from build123d import *

# Parameters (mm, degrees)
SKETCH2_W          = 40.136410409
SKETCH2_H          = 31
CUT_EXTRUDE1_DEPTH = 13
CUT_EXTRUDE3_START = -10
SKETCH4_R          = 3
CUT_EXTRUDE3_DEPTH = 73.147907447
SKETCH5_R          = 1.6
CUT_EXTRUDE4_DEPTH = 70.299079528
CIRPATTERN1_COUNT  = 3
CHAMFER1_SIZE      = 2.5
CHAMFER1_SIZE2     = 1.443375673


with BuildPart() as part:
    # Sketch1 → Revolve1 (revolve)
    with BuildSketch(Plane.XY):
        Polygon((-5.474803929, 60), (-33.724803929, 18), (-33.724803929, 0), (-22.724803929, 0), (-22.724803929, 13), (-3.474803929, 13), (-3.474803929, 60), align=None)
    revolve(axis=Axis((-2.724803929, 66.831705954, 0), (0, -1, 0)))

    # Sketch2 → Cut-Extrude1 (cut)
    with BuildSketch(Plane.XZ):
        with Locations((24.032962091, 0)):
            Rectangle(SKETCH2_W, SKETCH2_H)
    extrude(amount=-CUT_EXTRUDE1_DEPTH, mode=Mode.SUBTRACT)

    # Sketch4 → Cut-Extrude3 (cut)
    with BuildSketch(Plane(origin=(0, 18, 0), x_dir=(-1, 0, 0), z_dir=(0, 1, 0)).offset(CUT_EXTRUDE3_START)):
        with Locations(Location((27.724803929, 0, 0), (0, 0, 179.999995067))):
            Circle(SKETCH4_R)
    cut_extrude3 = extrude(amount=CUT_EXTRUDE3_DEPTH, mode=Mode.SUBTRACT)

    # Sketch5 → Cut-Extrude4 (cut, through all)
    with BuildSketch(Plane(origin=(0, 8, 0), x_dir=(1, 0, 0), z_dir=(0, 1, 0))):
        with Locations(Location((-27.724803929, 0, 0), (0, 0, 180))):
            Circle(SKETCH5_R)
    cut_extrude4 = extrude(amount=-CUT_EXTRUDE4_DEPTH, mode=Mode.SUBTRACT)

    # CirPattern1: Cut-Extrude3, Cut-Extrude4 ×3 about axis
    cirpattern1_axis = Axis((-2.724803929, 0, 0), (0, 1, 0))
    add([cut_extrude3.rotate(cirpattern1_axis, i * 360 / CIRPATTERN1_COUNT) for i in range(1, CIRPATTERN1_COUNT)], mode=Mode.SUBTRACT)
    add([cut_extrude4.rotate(cirpattern1_axis, i * 360 / CIRPATTERN1_COUNT) for i in range(1, CIRPATTERN1_COUNT)], mode=Mode.SUBTRACT)

    # Chamfer1
    chamfer1_edges = [part.edges().sort_by_distance(p)[0] for p in [
        (-1.974803929, 13, 0),
    ]]
    chamfer1_side = [part.faces().sort_by_distance(p)[0] for p in [
        (-1.974803929, 36.5, 0),
    ]]
    chamfer(chamfer1_edges, length=CHAMFER1_SIZE, length2=CHAMFER1_SIZE2, reference=chamfer1_side[0])


solid = part.part
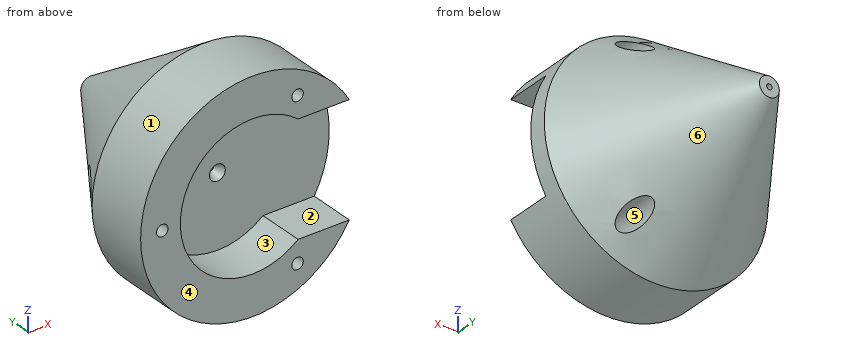
Here's how the part is built. I have some questions about the finished solid (model axes, mm). Face numbers are marked on the shaded views. A direction names the side the tool comes from. Round coordinates to 2 decimals unless told otherwise and drop trailing zeros. Order: outer loops, then holes, each group sorted by start corner. A loop starts at its lowest first (then second) coordinate and runs counter-clockwise, first axis right, second up. Notation, with made-up numbers: M 13.5,77.5 L 36.5,77.5 A20 ccw 36.5,86.5 Z; hole C -25.75,-10 d5. An arc over 180 degrees is marked long. One line per question, with ' | ' between items.
1) I'm going to push flat-ended pins straight in: pin 1 Ø4 at (x, y) = (18, 6) entering from +Z; pin 2 Ø4 at (x, z) = (-26.5, 23) entering from -Y; pin 3 Ø3 at (x, y) = (13, 15.5) entering from +Z; pin 4 Ø6.5 at (x, z) = (10.5, 20) entering from +Y. Where does each tip first touch, or does it pass through?
Checked values:
pin 1: stops at z = 24.71 | pin 2: passes through | pin 3: stops at z = 27.54 | pin 4: stops at y = 33.27
2) Imagine slicing it at C-C, the plane y = 50.5. Write out the boundary of the cut face in (x, z).
Checked values:
outline: C -2.72,0 d18.28; hole C -2.72,0 d1.5
3) On a 3-axis mill with a long thin cutter (end or side, diameter ignored), from which of +Z, -Z, +X, -X, +Y, -Y can I reach the whole of each face in a straight line? I mean the marked faces 1, 2 and 3. Say none if no direction works.
Checked values:
face 1: +Y, -Y | face 2: +X, -Y | face 3: -Y
4) We'd pull the mould along Z, two halves only. Please class the marked faces 4, 5 and 6: released by +Z, released by -Z, zero draft, split by the parting line, or undercut.
Checked values:
face 4: zero draft | face 5: undercut | face 6: split by the parting line
5) I need wall thicknesses on line 1 (Z direction, x = 10.5, y = 9); line 2 (X direction, y = 7.5, z = 18); line 3 (X direction, y = 3.5, z = 21). Which ranges of each line are inside material? Lowest first, please.
Checked values:
line 1: z = -28.04 to -24.56, -18.74 to -15.5, 15.5 to 18.74, 24.56 to 28.04 | line 2: x = -27.96 to -11.44, 5.99 to 22.51 | line 3: x = -25.53 to 8.31, 11.24 to 20.08
6) Imagine slicing it at A-A, the plane y = 25. Write out the boundary of the cut face in (x, z).
Checked values:
outline: M -28.87,-2.77 A26.29 ccw 7.95,-24.03 A3 cw long 12.75,-21.26 A26.29 ccw 12.75,21.26 A3 cw long 7.95,24.03 A26.29 ccw -28.87,2.77 A3 cw long Z; hole C -2.72,0 d1.5
7) Imagine slicing it at B-B, the plane y = 7. Write out the boundary of the cut face in (x, z).
Checked values:
outline: M 9.91,-15.5 A20 cw long 9.91,15.5 L 24.12,15.5 A31 ccw long 24.12,-15.5 Z; hole C -27.72,0 d3.2; hole C 9.78,-21.65 d3.2; hole C 9.78,21.65 d3.2
